Input: part model. Units: mm. Frame: model coordinates. Face numbers are marked on the shaded views. Coordinates: 2 decimals unless noted, no trailing zeros. Write each loop counter-clockwise with the first axis right and the second up, starting at its lowest first coordinate (ties: lowest second). Pieces come first, ordered by that corner, then holes. Notation, with made-up numbers: (51, -2) -> (85, -2) arc R18 cw to (85, 6) -> close; hole circle Ø10 at (-5, -4). An arc over 180 degrees is marked (long way). One line per question, with ' | ' between items. Start each with the question number.
```python
from build123d import *

# Parameters (mm, degrees)
SKETCH_1_W          = 4
SKETCH_1_H          = 68
EXTRUDE_1_DEPTH     = 300
FILLET_1_R          = 2
SKETCH_2_W          = 300
SKETCH_2_H          = 8
EXTRUDE_2_DEPTH     = 10
HOLE_WIZARD_M4_1_D  = 3.3
SKETCH_5_W          = 3
SKETCH_5_H          = 10
CUT_EXTRUDE_1_DEPTH = 62


with BuildPart() as part:
    # 草圖1 → 填料-伸長1 (new body)
    with BuildSketch(Plane(origin=(0, 0, 0), x_dir=(0, 0, -1), z_dir=(1, 0, 0))):
        Rectangle(SKETCH_1_W, SKETCH_1_H)
    extrude(amount=EXTRUDE_1_DEPTH)

    # 圓角1
    fillet_1_edges = [part.edges().sort_by_distance(p)[0] for p in [
        (150, -34, 2),
        (150, 34, 2),
    ]]
    fillet(fillet_1_edges, radius=FILLET_1_R)

    # 草圖2 → 填料-伸長2 (add)
    with BuildSketch(Plane(origin=(0, 0, -2), x_dir=(-1, 0, 0), z_dir=(0, 0, -1))):
        with Locations((-150, 27)):
            Rectangle(SKETCH_2_W, SKETCH_2_H)
        with Locations((-150, -27)):
            Rectangle(SKETCH_2_W, SKETCH_2_H)
    extrude(amount=EXTRUDE_2_DEPTH)

    # M4  螺絲攻的螺孔鑽1 (through all)
    with Locations(Plane(origin=(300, 0, 0), x_dir=(0, 0, -1), z_dir=(1, 0, 0))):
        with Locations((7, 26), (7, -26)):
            Hole(HOLE_WIZARD_M4_1_D / 2)

    # 草圖5 → 除料-伸長1 (cut)
    with BuildSketch(Plane(origin=(0, 31, 0), x_dir=(1, 0, 0), z_dir=(0, 1, 0))):
        with Locations((298.5, 7)):
            Rectangle(SKETCH_5_W, SKETCH_5_H)
    extrude(amount=-CUT_EXTRUDE_1_DEPTH, mode=Mode.SUBTRACT)


solid = part.part
```
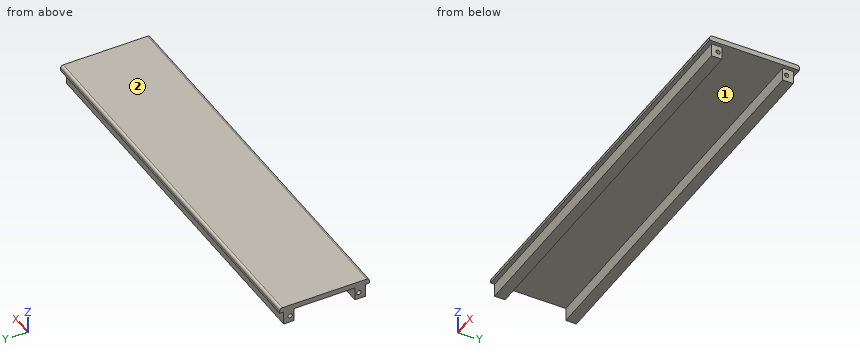
1) Section A-A, the plane x = 276. Return loops of the section in (y, z).
2) First-contact query: P1, Ø3, axis at x = 92.5, z = -5, coming from the -Y side; P2, Ø1.5, axis at y = -8.5, z = -4.5, coming from the +X side; P3, Ø2.5, axis at y = -28.5, z = -9, coming from the +X side; P4, Ø8, axis at x = 41.5, y = -17, coming from the -Z side. Flat tips, straight axial feed; report the tip coordinate or a pass-through.
3) Section B-B, the plane y = -1.5. Return loops of the section in (x, z), then the cut area to 3 significant figures.
4) Ray query, line 1 (Y direction, x = 154.5, z = -7); line 2 (Y direction, x = 174, z = -3.75); line 3 (Z direction, x = 65, y = 7). Return the intervals inside material, ascending.
5) Pull-direction query (Y, two-part tool) for the marked faces 1 and 2; classes: released by +Y, released by -Y, zero draft, split by the parting line, or undercut.
Answer block:
1) outline: (-34, -2) -> (-31, -2) -> (-31, -12) -> (-23, -12) -> (-23, -2) -> (23, -2) -> (23, -12) -> (31, -12) -> (31, -2) -> (34, -2) -> (34, 0) arc R2 ccw to (32, 2) -> (-32, 2) arc R2 ccw to (-34, 0) -> close; hole circle Ø3.3 at (-26, -7); hole circle Ø3.3 at (26, -7)
2) P1: stops at y = -31 | P2: passes through | P3: stops at x = 297 | P4: stops at z = -2
3) outline: (0, -2) -> (300, -2) -> (300, 2) -> (0, 2) -> close | area: 1,200 mm2
4) line 1: y = -31 to -27.65, -24.35 to -23, 23 to 24.35, 27.65 to 31 | line 2: y = -31 to -23, 23 to 31 | line 3: z = -2 to 2
5) face 1: undercut | face 2: zero draft
